Check sheet for the modelled part. Datum: model origin and axes. Units: mm. Face numbers are marked on the shaded views. A direction names the side the tool comes from. Give positions to 0.01 mm unless a question says otherwise; leave off trailing zeros. Order: outer loops, then holes, each group sorted by start corner. A loop starts at its lowest first (then second) coordinate and runs counter-clockwise, first axis right, second up. Notation, with made-up numbers: (79.25, -22) -> (102.25, -22) arc R14 ccw to (102.25, -10) -> close; hole circle Ø6 at (24, 56). An arc over 180 degrees is marked (long way). Answer in a Markdown table with one row per item. Add a question column.
(1) Thickness scan on L1, parallel to X at y = 67.5, z = 430; L2, parallel to Z at x = -3, y = 99; L3, parallel to Y at x = 12.5, z = 115.5. Record the ranges inside material, lowest first. Write a range as [from, to].
(2) Cross-section at D-D (z = 451.5). Record the cut outline in (x, y), then the cut area to 3 significant figures.
(3) Cross-section at B-B (y = 156). Record the cut outline in (x, z).
(4) Set-up check for the marked faces 1 and 2: record each of +Z, -Z, +X, -X, +Y, -Y from which the full face is reachable in a straight line by a thin tool's end or side.
(5) Go/stop test with flat-tipped pins: pin 1 (6 mm diameter, centred on x = -2.5, y = 81.5, fed in from -Z); pin 2 (5 mm diameter, centred on x = -5, z = 393, fed in from +Y); pin 3 (8 mm diameter, centred on x = 20.5, z = 141, fed in from +Y). Record where each tip stops, or that it passes through.
(6) Cross-section at C-C (z = 58.2). Record the cut outline in (x, y), then the cut area to 3 significant figures.
(7) Cross-section at A-A (y = 38). Record the cut outline in (x, z).
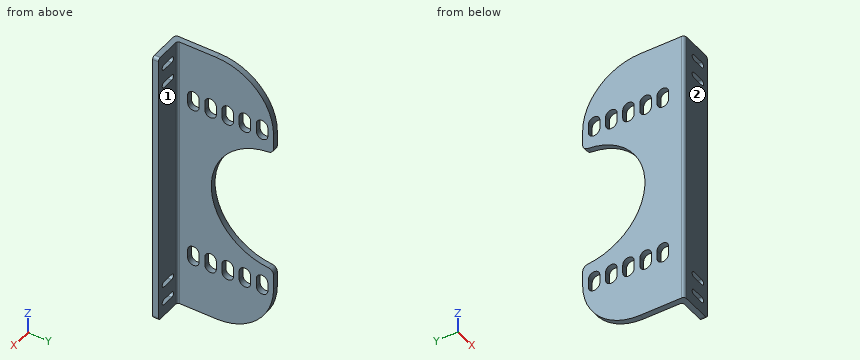
```python
from build123d import *

# Parameters (mm, degrees)
SZKIC1_W                    = 10
SZKIC1_H                    = 178
DODANIE_WYCI_GNI_CIE1_DEPTH = 490
WYTNIJ_WYCI_GNI_CIE1_DEPTH  = 522.424970633
WYTNIJ_WYCI_GNI_CIE2_DEPTH  = 522.424970633
ZAOKR_GLENIE1_R             = 100
ZAOKR_GLENIE2_R             = 100
WYTNIJ_WYCI_GNI_CIE3_DEPTH  = 522.424970633
ZAOKR_GLENIE3_R             = 10
SZKIC6_W                    = 60
SZKIC6_H                    = 10
DODANIE_WYCI_GNI_CIE2_DEPTH = 490
ZAOKR_GLENIE4_R             = 5
ZAOKR_GLENIE5_R             = 4
ZAOKR_GLENIE6_R             = 5
WYTNIJ_WYCI_GNI_CIE4_DEPTH  = 10
WYTNIJ_WYCI_GNI_CIE5_DEPTH  = 10


with BuildPart() as part:
    # Szkic1 → Dodanie-wyciągnięcie1 (new body)
    with BuildSketch(Plane.XY):
        with Locations((-5, 89)):
            Rectangle(SZKIC1_W, SZKIC1_H)
    extrude(amount=DODANIE_WYCI_GNI_CIE1_DEPTH)

    # Szkic2 → Wytnij-wyciągnięcie1 (cut, through all)
    with BuildSketch(Plane(origin=(0, 0, 0), x_dir=(0, 0, -1), z_dir=(1, 0, 0))):
        with BuildLine():
            Line((-107.5, 168), (-92.5, 168))
            ThreePointArc((-92.5, 168), (-82.5, 158), (-92.5, 148))
            Line((-92.5, 148), (-107.5, 148))
            ThreePointArc((-107.5, 148), (-117.5, 158), (-107.5, 168))
        make_face()
        with BuildLine():
            Line((-107.5, 138), (-92.5, 138))
            ThreePointArc((-92.5, 138), (-82.5, 128), (-92.5, 118))
            Line((-92.5, 118), (-107.5, 118))
            ThreePointArc((-107.5, 118), (-117.5, 128), (-107.5, 138))
        make_face()
        with BuildLine():
            Line((-107.5, 108), (-92.5, 108))
            ThreePointArc((-92.5, 108), (-82.5, 98), (-92.5, 88))
            Line((-92.5, 88), (-107.5, 88))
            ThreePointArc((-107.5, 88), (-117.5, 98), (-107.5, 108))
        make_face()
        with BuildLine():
            Line((-107.5, 78), (-92.5, 78))
            ThreePointArc((-92.5, 78), (-82.5, 68), (-92.5, 58))
            Line((-92.5, 58), (-107.5, 58))
            ThreePointArc((-107.5, 58), (-117.5, 68), (-107.5, 78))
        make_face()
        with BuildLine():
            Line((-107.5, 48), (-92.5, 48))
            ThreePointArc((-92.5, 48), (-82.5, 38), (-92.5, 28))
            Line((-92.5, 28), (-107.5, 28))
            ThreePointArc((-107.5, 28), (-117.5, 38), (-107.5, 48))
        make_face()
    extrude(amount=-WYTNIJ_WYCI_GNI_CIE1_DEPTH, mode=Mode.SUBTRACT)

    # Szkic3 → Wytnij-wyciągnięcie2 (cut, through all)
    with BuildSketch(Plane(origin=(0, 0, 0), x_dir=(0, 0, -1), z_dir=(1, 0, 0))):
        with BuildLine():
            Line((-397.5, 168), (-382.5, 168))
            ThreePointArc((-382.5, 168), (-372.5, 158), (-382.5, 148))
            Line((-382.5, 148), (-397.5, 148))
            ThreePointArc((-397.5, 148), (-407.5, 158), (-397.5, 168))
        make_face()
        with BuildLine():
            Line((-397.5, 138), (-382.5, 138))
            ThreePointArc((-382.5, 138), (-372.5, 128), (-382.5, 118))
            Line((-382.5, 118), (-397.5, 118))
            ThreePointArc((-397.5, 118), (-407.5, 128), (-397.5, 138))
        make_face()
        with BuildLine():
            Line((-397.5, 108), (-382.5, 108))
            ThreePointArc((-382.5, 108), (-372.5, 98), (-382.5, 88))
            Line((-382.5, 88), (-397.5, 88))
            ThreePointArc((-397.5, 88), (-407.5, 98), (-397.5, 108))
        make_face()
        with BuildLine():
            Line((-397.5, 78), (-382.5, 78))
            ThreePointArc((-382.5, 78), (-372.5, 68), (-382.5, 58))
            Line((-382.5, 58), (-397.5, 58))
            ThreePointArc((-397.5, 58), (-407.5, 68), (-397.5, 78))
        make_face()
        with BuildLine():
            Line((-397.5, 48), (-382.5, 48))
            ThreePointArc((-382.5, 48), (-372.5, 38), (-382.5, 28))
            Line((-382.5, 28), (-397.5, 28))
            ThreePointArc((-397.5, 28), (-407.5, 38), (-397.5, 48))
        make_face()
    extrude(amount=-WYTNIJ_WYCI_GNI_CIE2_DEPTH, mode=Mode.SUBTRACT)

    # Zaokrąglenie1
    zaokr_glenie1_edges = [part.edges().sort_by_distance(p)[0] for p in [
        (-5, 178, 0),
    ]]
    fillet(zaokr_glenie1_edges, radius=ZAOKR_GLENIE1_R)

    # Zaokrąglenie2
    zaokr_glenie2_edges = [part.edges().sort_by_distance(p)[0] for p in [
        (-5, 178, 490),
    ]]
    fillet(zaokr_glenie2_edges, radius=ZAOKR_GLENIE2_R)

    # Szkic5 → Wytnij-wyciągnięcie3 (cut, through all)
    with BuildSketch(Plane.ZY.offset(10)):
        with BuildLine():
            Line((136.235236097, 178), (353.764763903, 178))
            ThreePointArc((353.764763903, 178), (245, 69.235236097), (136.235236097, 178))
        make_face()
    extrude(amount=-WYTNIJ_WYCI_GNI_CIE3_DEPTH, mode=Mode.SUBTRACT)

    # Zaokrąglenie3
    zaokr_glenie3_edges = [part.edges().sort_by_distance(p)[0] for p in [
        (-5, 178, 353.764763903),
        (-5, 178, 136.235236097),
    ]]
    fillet(zaokr_glenie3_edges, radius=ZAOKR_GLENIE3_R)

    # Szkic6 → Dodanie-wyciągnięcie2 (add, through all)
    with BuildSketch(Plane(origin=(0, 0, 0), x_dir=(-1, 0, 0), z_dir=(0, 0, -1))):
        with Locations((-20, 5)):
            Rectangle(SZKIC6_W, SZKIC6_H)
    extrude(amount=-DODANIE_WYCI_GNI_CIE2_DEPTH)

    # Zaokrąglenie4
    zaokr_glenie4_edges = [part.edges().sort_by_distance(p)[0] for p in [
        (-10, 0, 245),
    ]]
    fillet(zaokr_glenie4_edges, radius=ZAOKR_GLENIE4_R)

    # Zaokrąglenie5
    zaokr_glenie5_edges = [part.edges().sort_by_distance(p)[0] for p in [
        (0, 10, 245),
    ]]
    fillet(zaokr_glenie5_edges, radius=ZAOKR_GLENIE5_R)

    # Zaokrąglenie6
    zaokr_glenie6_edges = [part.edges().sort_by_distance(p)[0] for p in [
        (50, 5, 0),
        (50, 5, 490),
    ]]
    fillet(zaokr_glenie6_edges, radius=ZAOKR_GLENIE6_R)

    # Szkic7 → Wytnij-wyciągnięcie4 (cut)
    with BuildSketch(Plane(origin=(0, 10, 0), x_dir=(1, 0, 0), z_dir=(0, 1, 0))):
        with BuildLine():
            Line((35, -470), (15, -470))
            ThreePointArc((15, -470), (10, -465), (15, -460))
            Line((15, -460), (35, -460))
            ThreePointArc((35, -460), (40, -465), (35, -470))
        make_face()
    wytnij_wyci_gni_cie4 = extrude(amount=-WYTNIJ_WYCI_GNI_CIE4_DEPTH, mode=Mode.SUBTRACT)

    # Lustro2: Wytnij-wyciągnięcie4 across plane
    add(wytnij_wyci_gni_cie4.mirror(Plane(origin=(0, 0, 245), x_dir=(1, 0, 0), z_dir=(0, 0, -1))), mode=Mode.SUBTRACT)

    # Szkic8 → Wytnij-wyciągnięcie5 (cut)
    with BuildSketch(Plane(origin=(0, 10, 0), x_dir=(1, 0, 0), z_dir=(0, 1, 0))):
        with BuildLine():
            Line((15, -426.8), (35, -426.8))
            ThreePointArc((35, -426.8), (40, -431.8), (35, -436.8))
            Line((35, -436.8), (15, -436.8))
            ThreePointArc((15, -436.8), (10, -431.8), (15, -426.8))
        make_face()
    wytnij_wyci_gni_cie5 = extrude(amount=-WYTNIJ_WYCI_GNI_CIE5_DEPTH, mode=Mode.SUBTRACT)

    # Lustro3: Wytnij-wyciągnięcie5 across plane
    add(wytnij_wyci_gni_cie5.mirror(Plane(origin=(0, 0, 245), x_dir=(1, 0, 0), z_dir=(0, 0, -1))), mode=Mode.SUBTRACT)


solid = part.part
```
Answer below:
| question | item | result |
|---|---|---|
| 1 | L1 | x = [-10, 0] |
| 1 | L2 | z = [2.23, 82.55], [117.45, 170.24], [319.76, 372.55], [407.45, 487.77] |
| 1 | L3 | y = [0, 10] |
| 2 | outline | (-10, 5) arc R5 ccw to (-5, 0) -> (50, 0) -> (50, 10) -> (4, 10) arc R4 cw to (0, 14) -> (0, 156.85) -> (-10, 156.85) -> close |
| 2 | area | 2,070 mm² |
| 3 | outline | (-10, 37.42) -> (0, 37.42) -> (0, 82.7) -> (-10, 82.7) -> close; (-10, 117.3) -> (0, 117.3) -> (0, 138.48) -> (-10, 138.48) -> close; (-10, 351.52) -> (0, 351.52) -> (0, 372.7) -> (-10, 372.7) -> close; (-10, 407.3) -> (0, 407.3) -> (0, 452.58) -> (-10, 452.58) -> close |
| 4 | face 1 | +Z, -Z, +X, +Y |
| 4 | face 2 | +Z, -Z, +X, -X, -Y |
| 5 | pin 1 | stops at z = 0 |
| 5 | pin 2 | stops at y = 178 |
| 5 | pin 3 | stops at y = 10 |
| 6 | outline | (-10, 5) arc R5 ccw to (-5, 0) -> (10, 0) -> (10, 10) -> (4, 10) arc R4 cw to (0, 14) -> (0, 168.84) -> (-10, 168.84) -> close; (40, 0) -> (50, 0) -> (50, 10) -> (40, 10) -> close |
| 6 | area | 1,890 mm² |
| 7 | outline | (-10, 0) -> (0, 0) -> (0, 82.5) -> (-10, 82.5) -> close; (-10, 117.5) -> (0, 117.5) -> (0, 372.5) -> (-10, 372.5) -> close; (-10, 407.5) -> (0, 407.5) -> (0, 490) -> (-10, 490) -> close |
